Source: CAD feature listing. Evaluate the final solid. Frame: model axes, mm. Face numbers are marked on the shaded views. A direction names the side the tool comes from. Give positions to 0.01 mm unless a question says otherwise; leave off trailing zeros. Write each loop counter-clockwise with the first axis right and the second up, starting at its lowest first coordinate (ties: lowest second). Pieces come first, ordered by that corner, then holes. Notation, with made-up numbers: (31.25, 85.5) -> (60.25, 85.5) arc R34 cw to (60.25, 116.5) -> close; hole circle Ø6 at (-14.75, 5). An arc over 180 degrees is marked (long way). Write item = value, one per line.
from build123d import *

# Parameters (mm, degrees)
SKETCH1_R           = 3.75
BOSS_EXTRUDE1_DEPTH = 30.5
SKETCH2_W           = 5.303300858
SKETCH2_H           = 5.303300858
BOSS_EXTRUDE2_DEPTH = 10
BOSS_EXTRUDE3_START = -10
BOSS_EXTRUDE3_DEPTH = 10


with BuildPart() as part:
    # Sketch1 → Boss-Extrude1 (new body)
    with BuildSketch(Plane(origin=(0, 0, 0), x_dir=(0, 0, -1), z_dir=(1, 0, 0))):
        Circle(SKETCH1_R)
    extrude(amount=-BOSS_EXTRUDE1_DEPTH)

    # Sketch2 → Boss-Extrude2 (add)
    with BuildSketch(Plane(origin=(0, 0, 0), x_dir=(0, 0, -1), z_dir=(1, 0, 0))):
        Rectangle(SKETCH2_W, SKETCH2_H)
    extrude(amount=BOSS_EXTRUDE2_DEPTH)

    # Sketch3 → Boss-Extrude3 (add)
    with BuildSketch(Plane.ZY.offset(30.5).offset(BOSS_EXTRUDE3_START)):
        with BuildLine():
            Line((-3.75, 0), (-3.75, 16))
            ThreePointArc((-3.75, 16), (0, 19.75), (3.75, 16))
            Line((3.75, 16), (3.75, 0))
            ThreePointArc((3.75, 0), (0, -3.75), (-3.75, 0))
        make_face()
    extrude(amount=BOSS_EXTRUDE3_DEPTH)


solid = part.part
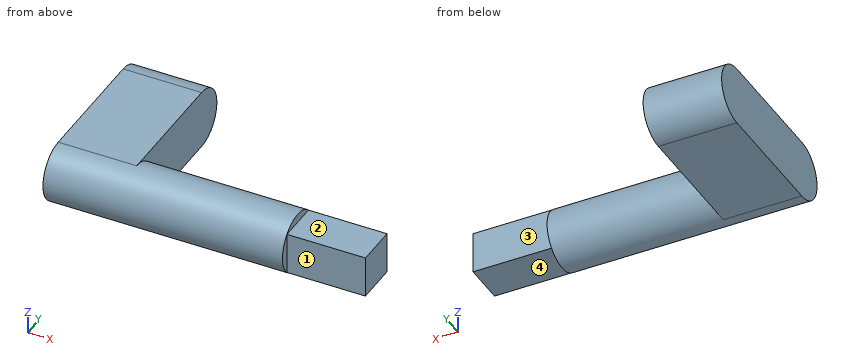
1) Cut plane D-D (y = 14). Return the cut outline in (x, z), then the cut area to 3 significant figures.
Computed:
outline = (-30.5, -3.75) -> (-20.5, -3.75) -> (-20.5, 3.75) -> (-30.5, 3.75) -> close
area = 75.0 mm²
2) Access query for the marked faces 1, 2, 3 and 4. Directions: +Z, -Z, +X, -X, +Y, -Y. A direction counts if a zero-diameter tool reaches every point of the face in a straight line with its end or side. Return the directions, or none.
Computed:
face_1 = +Z, -Z, +X, -Y
face_2 = +Z, +X, +Y, -Y
face_3 = +Z, -Z, +X, +Y
face_4 = -Z, +X, +Y, -Y
3) Cut plane B-B (y = 0.75). Return the cut outline in (x, z), then the cut area to 3 significant figures.
Computed:
outline = (-30.5, -3.75) -> (-20.5, -3.75) -> (-20.5, -3.67) -> (0, -3.67) -> (0, -2.65) -> (10, -2.65) -> (10, 2.65) -> (0, 2.65) -> (0, 3.67) -> (-20.5, 3.67) -> (-20.5, 3.75) -> (-30.5, 3.75) -> close
area = 279 mm²
4) Contact query for flat-ended pins moving along their axis: pin 1 (2 mm diameter, centred on y = 10.5, z = 0.5, fed in from +X); pin 2 (2.5 mm diameter, centred on x = 4, y = 0.5, fed in from +Z); pin 3 (12 mm diameter, centred on x = -4.5, y = 11.5, fed in from +Z); pin 4 (2 mm diameter, centred on x = -26, z = 2, fed in from -Y). Output: stop coordinate, or through.
Computed:
pin_1 = -20.5
pin_2 = 2.65
pin_3 = through
pin_4 = -3.61
5) Cut plane A-A (z = 0). Return the cut outline in (x, y), then the cut area to 3 significant figures.
Computed:
outline = (-30.5, -3.75) -> (0, -3.75) -> (0, -2.65) -> (10, -2.65) -> (10, 2.65) -> (0, 2.65) -> (0, 3.75) -> (-20.5, 3.75) -> (-20.5, 19.75) -> (-30.5, 19.75) -> close
area = 442 mm²
6) Material intervals for L1, parallel to X at y = 14.5, z = -2.5; L2, parallel to Z at x = 6, y = -0.5; L3, parallel to X at y = 0, z = -3, sorted ascending.
Computed:
L1 = -30.5 to -20.5
L2 = -2.65 to 2.65
L3 = -30.5 to 0
7) Cut plane C-C (x = -4.5). Return the cut outline in (y, z).
Computed:
outline = circle Ø7.5 at (0, 0)
